Geometry check sheet. Reference: the model listing, model coordinates, mm. A direction names the side the tool comes from. Give positions to 0.01 mm unless a question says otherwise; leave off trailing zeros. Order: outer loops, then holes, each group sorted by start corner. A loop starts at its lowest first (then second) coordinate and runs counter-clockwise, first axis right, second up.
from build123d import *

# Parameters (mm, degrees)
RESSALTO_EXTRUS_O1_DEPTH = 50
FILETE1_R                = 10


with BuildPart() as part:
    # Esboço1 → Ressalto-extrusão1 (new body)
    with BuildSketch(Plane.XY):
        Polygon((-10, 35), (-70, 35), (-70, -35), (70, -35), (70, 35), (40, 35), (40, 0), (-10, 0), align=None)
    extrude(amount=RESSALTO_EXTRUS_O1_DEPTH)

    # Filete1
    filete1_edges = [part.edges().sort_by_distance(p)[0] for p in [
        (-70, 35, 25),
    ]]
    fillet(filete1_edges, radius=FILETE1_R)


solid = part.part
Item 1: Sectioned sample at B-B (z = 46). Enter the section's corners in (x, y), and give its area (3 significant figures).
Reported:
outline: (-70, -35) - (70, -35) - (70, 35) - (40, 35) - (40, 0) - (-10, 0) - (-10, 35) - (-60, 35) arc R10 ccw to (-70, 25) - close
area: 8,030 mm2
Item 2: Sectioned sample at C-C (y = 30). Enter the section's corners in (x, z).
Reported:
outline: (-68.66, 0) - (-10, 0) - (-10, 50) - (-68.66, 50) - close; (40, 0) - (70, 0) - (70, 50) - (40, 50) - close
Item 3: Gauge pin test, flat end, axial feed: pin 1 (15 mm diameter, centred on x = 5, z = 24, fed in from +Y). Record the tip position at first contact, or that the pin passes through.
Reported:
pin 1: stops at y = 0
Item 4: Set-up check for faces 4 (the flat face through (70, 0, 25)), 5 (the flat face through (-10, 17, 25)): record each of +Z, -Z, +X, -X, +Y, -Y from which the full face is reachable in a straight line by a thin tool's end or side.
Reported:
face 4: +Z, -Z, +X, +Y, -Y
face 5: +Z, -Z, +Y
Item 5: Sectioned sample at A-A (y = 20). Enter the section's corners in (x, z).
Reported:
outline: (-70, 0) - (-10, 0) - (-10, 50) - (-70, 50) - close; (40, 0) - (70, 0) - (70, 50) - (40, 50) - close
Item 6: Draft check along X on faces 1 (the cylindrical face through (-66.99, 32.15, 25.35)), 2 (the flat face through (40, 18, 25)), 3 (the flat face through (-1, -7, 50)). Enter one of: released by +X, released by -X, zero draft, split by the parting line, or undercut.
Reported:
face 1: released by -X
face 2: undercut
face 3: zero draft
Item 7: Scan lines: L1, parallel to X at y = 5, z = 25; L2, parallel to Y at x = 32, z = 24.5; L3, parallel to X at y = 29.5, z = 31. Record each from-to range of solid material in increasing order.
Reported:
L1: x = -70 to -10, 40 to 70
L2: y = -35 to 0
L3: x = -68.93 to -10, 40 to 70
Item 8: Sectioned sample at D-D (x = 6). Enter the section's corners in (y, z).
Reported:
outline: (-35, 0) - (0, 0) - (0, 50) - (-35, 50) - close
